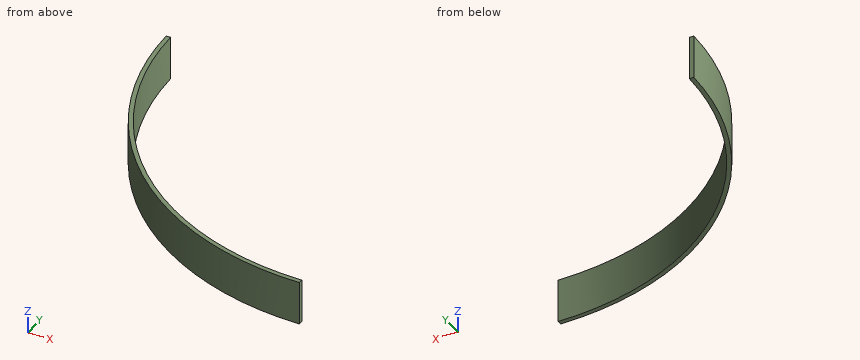
Autodesk Inventor part; units mm, degrees
ref_plane "YZ Plane" through (0, 0, 0) normal (1, 0, 0) x (0, 1, 0)
ref_plane "XZ Plane" through (0, 0, 0) normal (0, 1, 0) x (-1, 0, 0)
ref_plane "XY Plane" through (0, 0, 0) normal (0, 0, 1) x (1, 0, 0)
sketch "草圖1" plane through (0, 0, 0) normal (0, 0, 1) x (1, 0, 0)
  circle A0 centre (0, 0) radius 317
  circle A1 centre (0, 0) radius 322
  dimension "d0" = 634
  dimension "d1" = 644
extrude "擠出1" add sketch "草圖1" along normal blind 50
sketch "草圖2" plane through (0, 0, 50) normal (0, 0, 1) x (1, 0, 0)
  line L0 (-488.5314, 349.6941) -> (538.4038, 349.6941)
  line L1 (538.4038, 349.6941) -> (538.4038, 0)
  line L2 (538.4038, 0) -> (-488.5314, 0)
  line L3 (-488.5314, 0) -> (-488.5314, 349.6941)
  point P0 (0, 0)
  dimension "d4" = 0
extrude "擠出2" cut sketch "草圖2" against normal blind 50
sketch "草圖3" plane through (0, 0, 50) normal (0, 0, 1) x (1, 0, 0)
  line L0 (0, 139.236) -> (398.1663, 139.236)
  line L1 (398.1663, 139.236) -> (398.1663, -465.1236)
  line L2 (398.1663, -465.1236) -> (0, -465.1236)
  line L3 (0, -465.1236) -> (0, 139.236)
  point P0 (0, 0)
  dimension "d7" = 0
extrude "擠出3" cut sketch "草圖3" against normal blind 50
properties part number "鋁底板-半圓"
Geometry: final body of the model. Coordinates: model frame, mm. Round coordinates to 2 decimals unless told otherwise and drop trailing zeros. Order: outer loops, then holes, each group sorted by start corner. A loop starts at its lowest first (then second) coordinate and runs counter-clockwise, first axis right, second up. Notation, with made-up numbers: (-9, 16.25) -> (24, 16.25) arc R32 ccw to (24, 47.25) -> close; hole circle Ø10 at (3.5, 52.5). An arc over 180 degrees is marked (long way). Use one line per item in the form item = value.
(1) Section B-B on y = -64.5. Return loops of the section in (x, z), and give its area (3 significant figures).
Results list:
outline = (-315.47, 0) -> (-310.37, 0) -> (-310.37, 50) -> (-315.47, 50) -> close
area = 255 mm^2
(2) Ray query, probe 1 along Y at (x, z) = (-242, 6); probe 2 along X at (y, z) = (-171.5, 46.5); probe 3 along X at (y, z) = (-129.5, 24.5). Return the intervals inside material, ascending. Write a range as [from, to].
Results list:
probe_1 = [-212.41, -204.76]
probe_2 = [-272.53, -266.6]
probe_3 = [-294.81, -289.34]
(3) First-contact query: pin 1 Ø10 at (y, z) = (-48.5, 20) entering from +X; pin 2 Ø10 at (x, z) = (-87, 14) entering from -Y; pin 3 Ø3 at (x, z) = (-143.5, 39) entering from -Y. Flat tips, straight axial feed; report the tip coordinate or a pass-through.
Results list:
pin_1 = -312.45
pin_2 = -311.38
pin_3 = -289
(4) Section A-A on z = 36.5. Return loops of the section in (x, y), and give its area (3 significant figures).
Results list:
outline = (-322, 0) arc R322 ccw to (0, -322) -> (0, -317) arc R317 cw to (-317, 0) -> close
area = 2,510 mm^2
